Could you check a few things on this drawing? It's one solid part, dimensions in mm from its lowest x, y, z. Round coordinates to 2 decimals unless told otherwise and drop trailing zeros. Write each loop counter-clockwise with the first axis right and the second up, starting at its lowest first coordinate (ties: lowest second). Pieces come first, ordered by that corner, then holes. Notation, with made-up numbers: (-5.5, -33) - (8.5, -33) arc R35 cw to (8.5, 5) - close; hole circle Ø11 at (12.25, -2). An arc over 180 degrees is marked (long way). Write item = value, one per line. Start each with the question number.
Item 1: If I drill on line 1 along Y through (x, z) = (7, 0.6); line 2 along X through (y, z) = (69.5, 0.9); line 3 along X through (y, z) = (52.5, 0.6), over which ranges is the centre line in solid material (lowest first)? Write a range as [from, to].
Item 2: If we section it at A-A (x = 48.5): Please give me the cut outline in (y, z).
Item 3: If we section it at B-B (y = 34.5): Please give me the cut outline in (x, z).
Item 4: If we section it at D-D (z = 0.55): Please give me the cut outline in (x, y), and give its area (3 significant figures).
Item 5: If we section it at C-C (x = 7): Please give me the cut outline in (y, z).
Item 6: For P1, Ø0.6, axis at x = 27.5, z = 1, coming from the -Y side; P2, Ø5, axis at x = 7, y = 9.5, coming from the -Z side, each with a flat end and sliding along its axis, tell me the tip position at first contact or that it passes through.
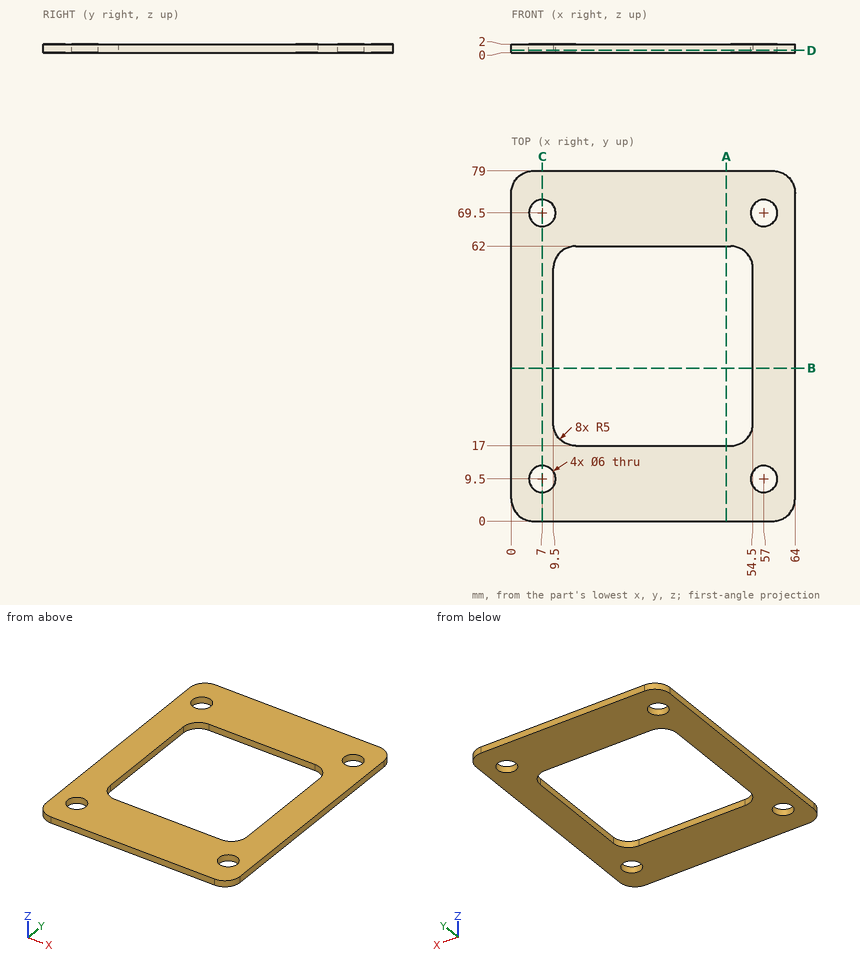
Reply:
q1.line_1 = [0, 6.5], [12.5, 66.5], [72.5, 79]
q1.line_2 = [0, 4], [10, 54], [60, 64]
q1.line_3 = [0, 9.5], [54.5, 64]
q2.outline = (0, 0) - (17, 0) - (17, 2) - (0, 2) - close; (62, 0) - (79, 0) - (79, 2) - (62, 2) - close
q3.outline = (0, 0) - (9.5, 0) - (9.5, 2) - (0, 2) - close; (54.5, 0) - (64, 0) - (64, 2) - (54.5, 2) - close
q4.outline = (0, 5) arc R5 ccw to (5, 0) - (59, 0) arc R5 ccw to (64, 5) - (64, 74) arc R5 ccw to (59, 79) - (5, 79) arc R5 ccw to (0, 74) - close; hole circle Ø6 at (7, 9.5); hole circle Ø6 at (7, 69.5); hole (9.5, 22) arc R5 ccw to (14.5, 17) - (49.5, 17) arc R5 ccw to (54.5, 22) - (54.5, 57) arc R5 ccw to (49.5, 62) - (14.5, 62) arc R5 ccw to (9.5, 57) - close; hole circle Ø6 at (57, 9.5); hole circle Ø6 at (57, 69.5)
q4.area = 2,920 mm2
q5.outline = (0, 0) - (6.5, 0) - (6.5, 2) - (0, 2) - close; (12.5, 0) - (66.5, 0) - (66.5, 2) - (12.5, 2) - close; (72.5, 0) - (79, 0) - (79, 2) - (72.5, 2) - close
q6.P1 = 0
q6.P2 = through
